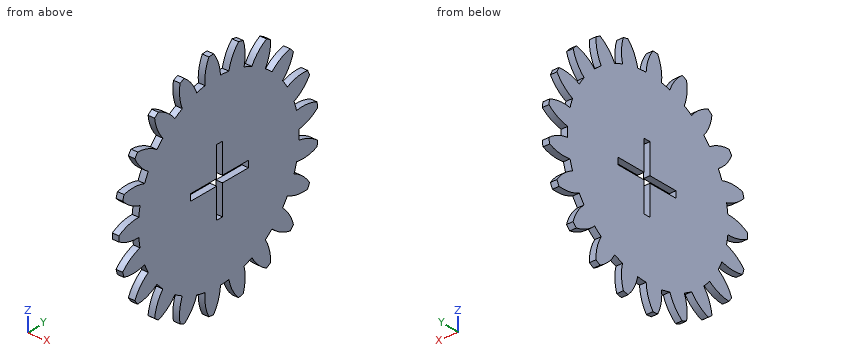
```python
from build123d import *

# Parameters (mm, degrees)
BASPROSKE_W        = 3
BASPROSKE_H        = 51.75
TOOTHCUT_DEPTH     = 74.247013591
TEETHCUTS_COUNT    = 21
TEETHCUTS_ANGLE    = 342.857142857
BORSKE_R           = 0.45
BORE_DEPTH         = 50.0000508
CUT_EXTRUDE1_DEPTH = 74.199531789


with BuildPart() as part:
    # BasProSke → Base-Revolve (revolve)
    with BuildSketch(Plane(origin=(0, 0, 0), x_dir=(1, 0, 0), z_dir=(0, 1, 0)), mode=Mode.PRIVATE) as base_revolve_sk:
        with Locations((1.5, 25.875)):
            Rectangle(BASPROSKE_W, BASPROSKE_H)
    revolve(base_revolve_sk.sketch.rotate(Axis((-10, 0, 0), (1, 0, 0)), 180), axis=Axis((-10, 0, 0), (1, 0, 0)))

    # TooCutSke → ToothCut (cut, through all)
    with BuildSketch(Plane(origin=(0, 0, 0), x_dir=(0, 0, -1), z_dir=(1, 0, 0))):
        with BuildLine():
            ThreePointArc((2.192126265, 41.566235798), (0, 41.624), (-2.192126265, 41.566235798))
            ThreePointArc((-2.192126265, 41.566235798), (-3.643354331, 46.777563157), (-6.511386997, 51.364325018))
            ThreePointArc((-6.511386997, 51.364325018), (0, 51.7754), (6.511386997, 51.364325018))
            ThreePointArc((6.511386997, 51.364325018), (3.643354331, 46.777563157), (2.192126265, 41.566235798))
        make_face()
    toothcut = extrude(amount=TOOTHCUT_DEPTH, mode=Mode.SUBTRACT)

    # TeethCuts: ToothCut ×21 about axis
    teethcuts_axis = Axis((-10, 0, 0), (1, 0, 0))
    for i in range(1, TEETHCUTS_COUNT):
        add(toothcut.rotate(teethcuts_axis, i * TEETHCUTS_ANGLE / (TEETHCUTS_COUNT - 1)), mode=Mode.SUBTRACT)

    # BorSke → Bore (cut, symmetric)
    with BuildSketch(Plane(origin=(0, 0, 0), x_dir=(0, 0, -1), z_dir=(1, 0, 0))):
        with Locations(Location((0, 0, 0), (0, 0, 180))):
            Circle(BORSKE_R)
    extrude(amount=BORE_DEPTH, both=True, mode=Mode.SUBTRACT)

    # Sketch1 → Cut-Extrude1 (cut, through all)
    with BuildSketch(Plane(origin=(3, 0, 0), x_dir=(0, 0, -1), z_dir=(1, 0, 0))):
        Polygon((1.5, 1.95), (15, 1.95), (15, -1.05), (1.5, -1.05), (1.5, -14.55), (-1.5, -14.55), (-1.5, -1.05), (-15, -1.05), (-15, 1.95), (-1.5, 1.95), (-1.5, 15.45), (1.5, 15.45), align=None)
    extrude(amount=-CUT_EXTRUDE1_DEPTH, mode=Mode.SUBTRACT)


solid = part.part
```
Geometry: final body of the model. Coordinates: model frame, mm. Coordinates: 2 decimals unless noted, no trailing zeros. Order: outer loops, then holes, each group sorted by start corner. A loop starts at its lowest first (then second) coordinate and runs counter-clockwise, first axis right, second up. Notation, with made-up numbers: (-22, 74) - (34, 74) arc R3 ccw to (34, 78) - close; hole circle Ø3 at (15, -13). An arc over 180 degrees is marked (long way). Write each question's results on one line, items separated by ' | '.
1) Line query: line 1 (Y direction, x = 2.1, z = -1); line 2 (Y direction, x = 1.9, z = 35); line 3 (Z direction, x = 1.3, y = -40.5). Output: solid intervals per line, ascending. Write a range as from..to.
Results list:
line 1: -51.74..-14.55, 15.45..41.61 | line 2: -32.02..-22.76, -22.53..24.84, 33.5..38.12 | line 3: -30.02..-23.5, -16.63..16.63, 23.5..30.02
2) Pin query (flat end, axial travel): pin 1 (1.5 mm diameter, centred on x = 2, z = 11.5, fed in from -Y); pin 2 (1.5 mm diameter, centred on x = 1, z = 0, fed in from +Y); pin 3 (1 mm diameter, centred on x = 0.5, z = -18, fed in from -Y). Return the tip coordinate at first contact, or that it passes through.
Results list:
pin 1: y = -47.97 | pin 2: y = 41.62 | pin 3: y = -37.77
3) Section B-B, the plane y = -26. Return loops of the section in (x, z).
Results list:
outline: (0, -38.28) - (3, -38.28) - (3, 38.28) - (0, 38.28) - close
4) Section A-A, the plane y = 3.5. Return loops of the section in (x, z).
Results list:
outline: (0, -41.48) - (3, -41.48) - (3, -1.5) - (0, -1.5) - close; (0, 1.5) - (3, 1.5) - (3, 41.48) - (0, 41.48) - close
